Here's how the part is built. I have some questions about the finished solid (model axes, mm). A direction names the side the tool comes from. Coordinates: 2 decimals unless noted, no trailing zeros. Loops run counter-clockwise (first coordinate to the right, second up) from the corner with the lowest first, then second, coordinate; pieces in that order, holes last. Notation, with made-up numbers: M 34,-25.75 L 82,-25.75 A16 cw 82,-2.75 Z; hole C 62.5,-11 d1. An arc over 180 degrees is marked long. Use CSV: the item, a comma, the result in double quotes. Start each with the question number.
Q1. For pin 1 Ø3 at (y, z) = (-33, -3.5) entering from +X; pin 2 Ø3 at (y, z) = (52, -2) entering from -X; pin 3 Ø2 at (x, y) = (-21, -40) entering from -Z, each with a flat end and sliding along its axis, tell me the tip position at first contact or that it passes through.
Q2. If we section it at B-B (y = 22): Please give me the cut outline in (x, z) (3 decimals), and give its area (3 significant figures).
Q3. Please list where these lines run through material, in increasing order: probe 1 along X at (y, z) = (-12.5, 0.25); probe 2 along X at (y, z) = (1, -2); probe 3 along Y at (x, z) = (12, -1.75) (3 decimals). Write a range as [from, to].
Q4. If we mould it in two halves opening along X, with no side actions, what happens to faces 1 (the cylindrical face through (16.31, -24.16, -3.22)), 2 (the flat face through (24.96, -60.325, -0.09)), 3 (the cylindrical face through (-34.923, 0.845, 0.14))? For each: +X half, -X half, draft (parallel to the pull), parting line (faces both ways), or undercut.
Q5. If we section it at C-C (x = -13): Please give me the cut outline in (y, z) (3 decimals), and give its area (3 significant figures).
Q6. If we section it at A-A (z = 1.75): State how many separate pieces and enclosed holes the cut face has, and give its area (3 significant figures).
Q7. Which directions (+Z, -Z, +X, -X, +Y, -Y) give clear straight access to the entire face, cutting with the end or side of a thin tool? Please do faces 4 (the cylindrical face through (-20.525, 33.774, -3.219)), 5 (the flat face through (0, 1, 6.35)), 6 (the cylindrical face through (6.856, 45.174, 0.089)), 7 (the cylindrical face through (-19.556, -48.349, 0.089)), 8 (the flat face through (-20, -32, 0)).
from build123d import *

# Parameters (mm, degrees)
SKETCH1_R               = 3.429
BOSS_EXTRUDE1_DEPTH     = 60.325
CUT_EXTRUDE1_DEPTH      = 70.9941694
CUT_EXTRUDE1_DEPTH_BACK = 70.9941694
FILLET1_R               = 2.54
CUT_EXTRUDE3_DEPTH      = 71.853025694
CUT_EXTRUDE3_DEPTH_BACK = 71.853025694
SKETCH5_W               = 40.64
SKETCH5_H               = 12.7
FILLET2_R               = 2.54
SKETCH4_R               = 1.984375
CUT_EXTRUDE2_DEPTH      = 6.35
SKETCH6_R               = 1.984375
CUT_EXTRUDE4_DEPTH      = 6.35
SKETCH7_R               = 1.984375
CUT_EXTRUDE5_DEPTH      = 6.35


with BuildPart() as part:
    # Sketch1 → Boss-Extrude1 (new, symmetric)
    with BuildSketch(Plane(origin=(0, 0, 0), x_dir=(1, 0, 0), z_dir=(0, 1, 0))):
        with BuildLine():
            Line((-28.575, 6.35), (28.575, 6.35))
            ThreePointArc((28.575, 6.35), (34.925, 0), (28.575, -6.35))
            Line((28.575, -6.35), (-28.575, -6.35))
            ThreePointArc((-28.575, -6.35), (-34.925, 0), (-28.575, 6.35))
        make_face()
        with Locations(Location((28.575, 0, 0), (0, 0, 90))):
            Circle(SKETCH1_R, mode=Mode.SUBTRACT)
        with Locations(Location((-28.575, 0, 0), (0, 0, 90))):
            Circle(SKETCH1_R, mode=Mode.SUBTRACT)
    extrude(amount=BOSS_EXTRUDE1_DEPTH, both=True)

    # Sketch2 → Cut-Extrude1 (cut, two sides: drawn at the far end of the back side and taken through both)
    with BuildSketch(Plane.XY.offset(-CUT_EXTRUDE1_DEPTH_BACK)):
        Polygon((-7.62, 326.18824101), (-7.62, 60.325), (-7.62, 44.45), (7.62, 44.45), (7.62, 60.325), (7.62, 326.18824101), (7.62, 857.914723029), (-7.62, 857.914723029), align=None)
    extrude(amount=CUT_EXTRUDE1_DEPTH + CUT_EXTRUDE1_DEPTH_BACK, mode=Mode.SUBTRACT)

    # Fillet1
    fillet1_edges = [part.edges().sort_by_distance(p)[0] for p in [
        (-7.62, 44.45, 0),
        (7.62, 44.45, 0),
        (7.62, 60.325, 0),
        (-7.62, 60.325, 0),
    ]]
    fillet(fillet1_edges, radius=FILLET1_R)

    # Sketch5 → Cut-Extrude3 (cut, two sides: drawn at the far end of the back side and taken through both)
    with BuildSketch(Plane.XY.offset(6.35).offset(-CUT_EXTRUDE3_DEPTH_BACK)):
        with Locations((0, -53.975)):
            Rectangle(SKETCH5_W, SKETCH5_H)
    extrude(amount=CUT_EXTRUDE3_DEPTH + CUT_EXTRUDE3_DEPTH_BACK, mode=Mode.SUBTRACT)

    # Fillet2
    fillet2_edges = [part.edges().sort_by_distance(p)[0] for p in [
        (-20.32, -60.325, 0),
        (-20.32, -47.625, 0),
        (20.32, -47.625, 0),
        (20.32, -60.325, 0),
    ]]
    fillet(fillet2_edges, radius=FILLET2_R)

    # Sketch4 → Cut-Extrude2 (cut)
    with BuildSketch(Plane.XY.offset(6.35)):
        with Locations((-6.985, -6.985)):
            Circle(SKETCH4_R)
        with Locations((-19.685, -32.385)):
            Circle(SKETCH4_R)
    extrude(amount=-CUT_EXTRUDE2_DEPTH, mode=Mode.SUBTRACT)

    # Sketch6 → Cut-Extrude4 (cut)
    with BuildSketch(Plane(origin=(0, 0, -6.35), x_dir=(-1, 0, 0), z_dir=(0, 0, -1))):
        with Locations((5.08, 35.711069013)):
            Circle(SKETCH6_R)
        with Locations((20.955, 35.711069013)):
            Circle(SKETCH6_R)
        with Locations((5.08, -40.488930987)):
            Circle(SKETCH6_R)
        with Locations((20.955, -40.488930987)):
            Circle(SKETCH6_R)
    extrude(amount=-CUT_EXTRUDE4_DEPTH, mode=Mode.SUBTRACT)

    # Sketch7 → Cut-Extrude5 (cut)
    with BuildSketch(Plane(origin=(0, 0, -6.35), x_dir=(-1, 0, 0), z_dir=(0, 0, -1))):
        with Locations((-15.875, 15.875)):
            Circle(SKETCH7_R)
        with Locations((-15.875, -22.225)):
            Circle(SKETCH7_R)
    extrude(amount=-CUT_EXTRUDE5_DEPTH, mode=Mode.SUBTRACT)


solid = part.part
Results below:
1,pin 1,"x = 34.6"
1,pin 2,"x = -34.91"
1,pin 3,"z = 0"
2,outline,"M -28.575,-6.35 L 28.575,-6.35 A6.35 ccw 28.575,6.35 L -28.575,6.35 A6.35 ccw Z; hole C -28.575,0 d6.858; hole C 28.575,0 d6.858"
2,area,"779 mm^2"
3,probe 1,"[-34.92, -31.99], [-25.16, 25.16], [31.99, 34.92]"
3,probe 2,"[-34.6, -31.36], [-25.79, 25.79], [31.36, 34.6]"
3,probe 3,"[-47.625, 60.325]"
4,face 1,"undercut"
4,face 2,"draft"
4,face 3,"-X half"
5,outline,"M -47.625,-6.35 L 60.325,-6.35 L 60.325,6.35 L -47.625,6.35 Z"
5,area,"1,370 mm^2"
6,separate pieces,"3"
6,enclosed holes,"2"
6,area,"6,160 mm^2"
7,face 4,"-Z"
7,face 5,"+Z, +X, -X, +Y, -Y"
7,face 6,"+Z, -Z, +Y"
7,face 7,"+Z, -Z, -Y"
7,face 8,"+Z"
